```python
from build123d import *

# Parameters (mm, degrees)
SKETCH1_R       = 3.35
EXTRUSION_DEPTH = 100


with BuildPart() as part:
    # Sketch1 → Extrusion (new body)
    with BuildSketch(Plane(origin=(0, 0, 0), x_dir=(1, 0, 0), z_dir=(0, 1, 0))):
        with BuildLine():
            Line((14.1, -4), (13.9, -4))
            ThreePointArc((13.9, -4), (13.263603897, -4.263603897), (13, -4.9))
            Line((13, -4.9), (13, -8.985786438))
            ThreePointArc((13, -8.985786438), (12.382683432, -9.90966597), (11.292893219, -9.692893219))
            Line((11.292893219, -9.692893219), (5.835786438, -4.235786438))
            ThreePointArc((5.835786438, -4.235786438), (5.402240935, -3.58693974), (5.25, -2.821572875))
            Line((5.25, -2.821572875), (5.25, 2.821572875))
            ThreePointArc((5.25, 2.821572875), (5.402240935, 3.58693974), (5.835786438, 4.235786438))
            Line((5.835786438, 4.235786438), (11.292893219, 9.692893219))
            ThreePointArc((11.292893219, 9.692893219), (12.382683432, 9.90966597), (13, 8.985786438))
            Line((13, 8.985786438), (13, 4.9))
            ThreePointArc((13, 4.9), (13.263603897, 4.263603897), (13.9, 4))
            Line((13.9, 4), (14.1, 4))
            ThreePointArc((14.1, 4), (14.736396103, 4.263603897), (15, 4.9))
            Line((15, 4.9), (15, 13))
            ThreePointArc((15, 13), (14.414213562, 14.414213562), (13, 15))
            Line((13, 15), (4.9, 15))
            ThreePointArc((4.9, 15), (4.263603897, 14.736396103), (4, 14.1))
            Line((4, 14.1), (4, 13.9))
            ThreePointArc((4, 13.9), (4.263603897, 13.263603897), (4.9, 13))
            Line((4.9, 13), (8.985786438, 13))
            ThreePointArc((8.985786438, 13), (9.90966597, 12.382683432), (9.692893219, 11.292893219))
            Line((9.692893219, 11.292893219), (4.235786438, 5.835786438))
            ThreePointArc((4.235786438, 5.835786438), (3.58693974, 5.402240935), (2.821572875, 5.25))
            Line((2.821572875, 5.25), (-2.821572875, 5.25))
            ThreePointArc((-2.821572875, 5.25), (-3.58693974, 5.402240935), (-4.235786438, 5.835786438))
            Line((-4.235786438, 5.835786438), (-9.692893219, 11.292893219))
            ThreePointArc((-9.692893219, 11.292893219), (-9.90966597, 12.382683432), (-8.985786438, 13))
            Line((-8.985786438, 13), (-4.9, 13))
            ThreePointArc((-4.9, 13), (-4.263603897, 13.263603897), (-4, 13.9))
            Line((-4, 13.9), (-4, 14.1))
            ThreePointArc((-4, 14.1), (-4.263603897, 14.736396103), (-4.9, 15))
            Line((-4.9, 15), (-13, 15))
            ThreePointArc((-13, 15), (-14.414213562, 14.414213562), (-15, 13))
            Line((-15, 13), (-15, 4.9))
            ThreePointArc((-15, 4.9), (-14.736396103, 4.263603897), (-14.1, 4))
            Line((-14.1, 4), (-13.9, 4))
            ThreePointArc((-13.9, 4), (-13.263603897, 4.263603897), (-13, 4.9))
            Line((-13, 4.9), (-13, 8.985786438))
            ThreePointArc((-13, 8.985786438), (-12.382683432, 9.90966597), (-11.292893219, 9.692893219))
            Line((-11.292893219, 9.692893219), (-5.835786438, 4.235786438))
            ThreePointArc((-5.835786438, 4.235786438), (-5.402240935, 3.58693974), (-5.25, 2.821572875))
            Line((-5.25, 2.821572875), (-5.25, -2.821572875))
            ThreePointArc((-5.25, -2.821572875), (-5.402240935, -3.58693974), (-5.835786438, -4.235786438))
            Line((-5.835786438, -4.235786438), (-11.292893219, -9.692893219))
            ThreePointArc((-11.292893219, -9.692893219), (-12.382683432, -9.90966597), (-13, -8.985786438))
            Line((-13, -8.985786438), (-13, -4.9))
            ThreePointArc((-13, -4.9), (-13.263603897, -4.263603897), (-13.9, -4))
            Line((-13.9, -4), (-14.1, -4))
            ThreePointArc((-14.1, -4), (-14.736396103, -4.263603897), (-15, -4.9))
            Line((-15, -4.9), (-15, -13))
            ThreePointArc((-15, -13), (-14.414213562, -14.414213562), (-13, -15))
            Line((-13, -15), (-4.9, -15))
            ThreePointArc((-4.9, -15), (-4.263603897, -14.736396103), (-4, -14.1))
            Line((-4, -14.1), (-4, -13.9))
            ThreePointArc((-4, -13.9), (-4.263603897, -13.263603897), (-4.9, -13))
            Line((-4.9, -13), (-8.985786438, -13))
            ThreePointArc((-8.985786438, -13), (-9.90966597, -12.382683432), (-9.692893219, -11.292893219))
            Line((-9.692893219, -11.292893219), (-4.235786438, -5.835786438))
            ThreePointArc((-4.235786438, -5.835786438), (-3.58693974, -5.402240935), (-2.821572875, -5.25))
            Line((-2.821572875, -5.25), (2.821572875, -5.25))
            ThreePointArc((2.821572875, -5.25), (3.58693974, -5.402240935), (4.235786438, -5.835786438))
            Line((4.235786438, -5.835786438), (9.692893219, -11.292893219))
            ThreePointArc((9.692893219, -11.292893219), (9.90966597, -12.382683432), (8.985786438, -13))
            Line((8.985786438, -13), (4.9, -13))
            ThreePointArc((4.9, -13), (4.263603897, -13.263603897), (4, -13.9))
            Line((4, -13.9), (4, -14.1))
            ThreePointArc((4, -14.1), (4.263603897, -14.736396103), (4.9, -15))
            Line((4.9, -15), (13, -15))
            ThreePointArc((13, -15), (14.414213562, -14.414213562), (15, -13))
            Line((15, -13), (15, -4.9))
            ThreePointArc((15, -4.9), (14.736396103, -4.263603897), (14.1, -4))
        make_face()
        Circle(SKETCH1_R, mode=Mode.SUBTRACT)
    extrude(amount=-EXTRUSION_DEPTH)


solid = part.part
```
Could you check a few things on this model? Use its own coordinates, in mm. A direction names the side the tool comes from. Coordinates: 2 decimals unless noted, no trailing zeros. Loops run counter-clockwise (first coordinate to the right, second up) from the corner with the lowest first, then second, coordinate; pieces in that order, holes last. Notation, with made-up numbers: M 77,30 L 123,30 A11 cw 123,44 Z; hole C 69.5,66.25 d6. An arc over 180 degrees is marked long. Put each result on its own line as item: value. Start each with the question number.
(1) Thinking about a two-plate mould opening in Z: for faces 1 (the face through (-15, -49, -9)), 2 (the face through (0, -49, -5.25)), 3 (the face through (-7, -49, -13)), 4 (the face through (-9, -49, 15)), which applies, pulls with the +Z half, pulls with the -Z half, needs draft (parallel to the pull), parting line crosses it, or undercut?
(2) Suppose I cut it at C-C on x = 0. Please give me the cut outline in (y, z), then the cut area to 3 significant figures.
(3) I need wall thicknesses on line 1 (X direction, y = -55, z = 0); line 2 (X direction, y = -51, z = -7.25); line 3 (X direction, y = -78.5, z = -9.25). Which ranges of each line are inside material? Lowest first, please. Write a range as from..to.
(4) For faces 5 (the face through (-9.903, -49.3, 12.398)), 6 (the face through (9, -49, -15)), which set-ups out of +Z, -Z, +X, -X, +Y, -Y let a thin tool reach every point of the face, with its end or its side?
(5) Will these pins go through, and if not, where does the flat tip stop? P1, Ø3, axis at x = -2, y = -14, coming from the +Z side; P2, Ø4.5, axis at x = 0, y = -40.5, coming from the -Z side.
(6) Suppose I cut it at A-A on x = -6.75. Please give me the cut outline in (y, z), then the cut area to 3 significant figures.
(7) Suppose I cut it at B-B on z = 0. Please give me the cut outline in (x, y).
Solutions:
1. face 1: needs draft
1. face 2: pulls with the -Z half
1. face 3: undercut
1. face 4: pulls with the +Z half
2. outline: M -100,-5.25 L 0,-5.25 L 0,-3.35 L -100,-3.35 Z; M -100,3.35 L 0,3.35 L 0,5.25 L -100,5.25 Z
2. area: 380 mm2
3. line 1: x = -5.25..-3.35, 3.35..5.25
3. line 2: x = -15..-13, -8.85..-5.65, 5.65..8.85, 13..15
3. line 3: x = -15..-12.96, -10.85..-7.65, 7.65..10.85, 12.96..15
4. face 5: +Y, -Y
4. face 6: -Z, +X, -X, +Y, -Y
5. P1: stops at z = 5.37
5. P2: stops at z = -5.25
6. outline: M -100,-15 L 0,-15 L 0,-13 L -100,-13 Z; M -100,-8.35 L 0,-8.35 L 0,-5.15 L -100,-5.15 Z; M -100,5.15 L 0,5.15 L 0,8.35 L -100,8.35 Z; M -100,13 L 0,13 L 0,15 L -100,15 Z
6. area: 1,040 mm2
7. outline: M -5.25,-100 L -3.35,-100 L -3.35,0 L -5.25,0 Z; M 3.35,-100 L 5.25,-100 L 5.25,0 L 3.35,0 Z
